```python
from build123d import *

# Parameters (mm, degrees)
SKETCH1_R           = 10.25
SKETCH1_R_2         = 2.75
BOSS_EXTRUDE1_DEPTH = 4
CHAMFER1_SIZE       = 0.5


with BuildPart() as part:
    # Sketch1 → Boss-Extrude1 (new body)
    with BuildSketch(Plane(origin=(0, 0, 0), x_dir=(1, 0, 0), z_dir=(0, 1, 0))):
        with BuildLine():
            Line((-11, 18), (11, 18))
            ThreePointArc((11, 18), (15.949747468, 15.949747468), (18, 11))
            Line((18, 11), (18, -11))
            ThreePointArc((18, -11), (15.949747468, -15.949747468), (11, -18))
            Line((11, -18), (-11, -18))
            ThreePointArc((-11, -18), (-15.949747468, -15.949747468), (-18, -11))
            Line((-18, -11), (-18, 11))
            ThreePointArc((-18, 11), (-15.949747468, 15.949747468), (-11, 18))
        make_face()
        Circle(SKETCH1_R, mode=Mode.SUBTRACT)
        with Locations((-11.525840533, 11.525840533)):
            Circle(SKETCH1_R_2, mode=Mode.SUBTRACT)
        with Locations((11.525840533, 11.525840533)):
            Circle(SKETCH1_R_2, mode=Mode.SUBTRACT)
        with Locations((11.525840533, -11.525840533)):
            Circle(SKETCH1_R_2, mode=Mode.SUBTRACT)
        with Locations((-11.525840533, -11.525840533)):
            Circle(SKETCH1_R_2, mode=Mode.SUBTRACT)
    extrude(amount=BOSS_EXTRUDE1_DEPTH)

    # Chamfer1
    chamfer1_edges = [part.edges().sort_by_distance(p)[0] for p in [
        (18, 0, 0),
        (15.949747468, 0, 15.949747468),
        (0, 0, 18),
        (-15.949747468, 0, 15.949747468),
        (15.949747468, 4, 15.949747468),
        (18, 4, 0),
        (15.949747468, 4, -15.949747468),
        (-10.25, 0, 0),
        (-10.25, 4, 0),
        (0, 4, -18),
        (-14.275840533, 0, -11.525840533),
        (-14.275840533, 4, -11.525840533),
        (-15.949747468, 4, -15.949747468),
        (8.775840533, 0, -11.525840533),
        (8.775840533, 4, -11.525840533),
        (-18, 4, 0),
        (8.775840533, 0, 11.525840533),
        (8.775840533, 4, 11.525840533),
        (-14.275840533, 0, 11.525840533),
        (-14.275840533, 4, 11.525840533),
        (-15.949747468, 4, 15.949747468),
        (-18, 0, 0),
        (0, 4, 18),
        (-15.949747468, 0, -15.949747468),
        (0, 0, -18),
        (15.949747468, 0, -15.949747468),
    ]]
    chamfer(chamfer1_edges, length=CHAMFER1_SIZE)


solid = part.part
```
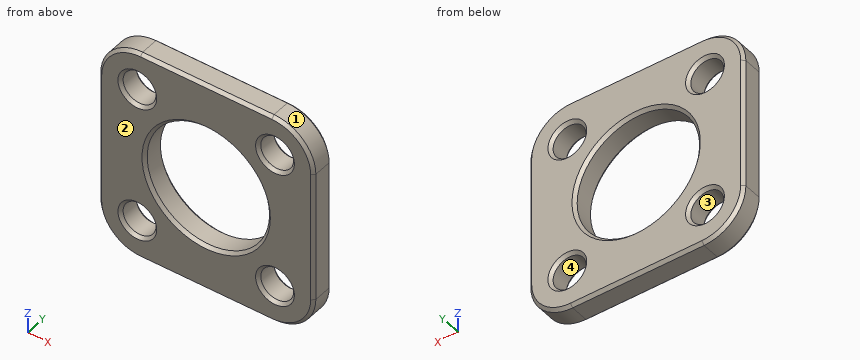
Geometry check sheet. Reference: the model listing, model coordinates, mm. Face numbers are marked on the shaded views. Coordinates: 2 decimals unless noted, no trailing zeros. Order: outer loops, then holes, each group sorted by start corner. A loop starts at its lowest first (then second) coordinate and runs counter-clockwise, first axis right, second up.
Item 1: Section check A-A (z = 0). Enter the section's corners in (x, y).
Item 2: Section check C-C (x = -11.5). Count the separate pieces of the cut face and the enclosed holes in it, plus the area to 3 significant figures.
Item 3: Scan lines: line 1 along X through (y, z) = (0.35, 11.5); line 2 along Z through (x, y) = (10.5, 1.5); line 3 along Z through (x, y) = (9, 2.5). Record each from-to range of solid material in increasing order.
Item 4: Section check B-B (y = 2.85). Enter the section's corners in (x, z).
Item 5: Mould release check, pull along Z, two halves, no side actions. Record for the marked faces 1, 2, 3 and 4: released by +Z, released by -Z, zero draft, split by the parting line, or undercut.
Item 6: Depth check by flat-ended pin: pin 1 (4.5 mm diameter, centred on x = 11.53, z = -11.53, fed in from -Y). Enter the tip coordinate at first touch or a pass-through.
Check sheet entries:
1. outline: (-18, 0.5) - (-17.5, 0) - (-10.75, 0) - (-10.25, 0.5) - (-10.25, 3.5) - (-10.75, 4) - (-17.5, 4) - (-18, 3.5) - close; (10.25, 0.5) - (10.75, 0) - (17.5, 0) - (18, 0.5) - (18, 3.5) - (17.5, 4) - (10.75, 4) - (10.25, 3.5) - close
2. separate pieces: 3
2. enclosed holes: 0
2. area: 98.4 mm2
3. line 1: x = -17.83 to -14.43, -8.63 to 8.63, 14.43 to 17.83
3. line 2: z = -18 to -14.08, -8.97 to 8.97, 14.08 to 18
3. line 3: z = -18 to -12.61, -10.44 to -4.91, 4.91 to 10.44, 12.61 to 18
4. outline: (-18, -11) arc R7 ccw to (-11, -18) - (11, -18) arc R7 ccw to (18, -11) - (18, 11) arc R7 ccw to (11, 18) - (-11, 18) arc R7 ccw to (-18, 11) - close; hole circle Ø5.5 at (-11.53, -11.53); hole circle Ø5.5 at (-11.53, 11.53); hole circle Ø20.5 at (0, 0); hole circle Ø5.5 at (11.53, -11.53); hole circle Ø5.5 at (11.53, 11.53)
5. face 1: released by +Z
5. face 2: zero draft
5. face 3: undercut
5. face 4: undercut
6. pin 1: passes through
